Part model, mm, in its own coordinate system. A direction names the side the tool comes from. Coordinates: 2 decimals unless noted, no trailing zeros. Write each loop counter-clockwise with the first axis right and the second up, starting at its lowest first coordinate (ties: lowest second). Pieces come first, ordered by that corner, then holes. Notation, with made-up numbers: (26.5, 80) - (38.5, 80) arc R28 ccw to (38.5, 110) - close; hole circle Ø10 at (78.5, -2). An arc over 180 degrees is marked (long way). Use one line per item in the form item = value. Start each with the question number.
Autodesk Inventor part; units mm, degrees
ref_plane "YZ Plane" through (0, 0, 0) normal (1, 0, 0) x (0, 1, 0)
ref_plane "XZ Plane" through (0, 0, 0) normal (0, 1, 0) x (-1, 0, 0)
ref_plane "XY Plane" through (0, 0, 0) normal (0, 0, 1) x (1, 0, 0)
sketch "Sketch1" plane through (0, 0, 0) normal (0, 1, 0) x (-1, 0, 0)
  line L0 (-20, 40) -> (20, 40)
  line L1 (20, 40) -> (20, -40)
  line L2 (20, -40) -> (-20, -40)
  line L3 (-20, -40) -> (-20, 40)
  arc A0 (20, 14.9917) -> (20, -14.9917) centre (20.5, 0) ccw
  point P0 (0, 0)
  dimension "d0" = 80
  dimension "d1" = 40
  dimension "d2" = 40
  dimension "d3" = 20
  dimension "d4" = 30
  dimension "d22" = 0.5
extrude "Extrusion1" add sketch "Sketch1" along normal blind 20 contours L0 L1 A0 L2 L3
sketch "Sketch2" plane through (20, 0, 40) normal (1, 0, 0) x (0, 0, -1)
  line L0 (0, 0) -> (80, 0)
  line L1 (80, 0) -> (80, 20)
  line L2 (0, 20) -> (80, 20)
  line L3 (0, 0) -> (0, 20)
  point P0 (40, 0)
  point P1 (10, 10)
  point P2 (70, 10)
  dimension "d8" = 10
  dimension "d9" = 10
  dimension "d10" = 10
  dimension "d11" = 10
hole "Hole1" at (20, 10, 30) at (20, 10, -30) direction (-1, 0, 0) diameter 6 end through all
sketch "Sketch3" plane through (0, 20, 0) normal (0, 1, 0) x (1, 0, 0)
  line L0 (20, -40) -> (20, 40)
  line L1 (20, 40) -> (-20, 40)
  line L2 (-20, 40) -> (-20, 14.9917)
  arc A0 (-20, -14.9917) -> (-20, 14.9917) centre (-20.5, 0) ccw
  line L3 (-20, -14.9917) -> (-20, -40)
  line L4 (-20, -40) -> (20, -40)
  line L5 (20, -17.75) -> (2.75, -17.75)
  line L6 (2.75, -17.75) -> (2.75, 17.75)
  line L7 (2.75, 17.75) -> (20, 17.75)
  point P0 (0, 0)
  dimension "d19" = 17.25
  dimension "d20" = 35.5
  dimension "d21" = 17.75
extrude "Extrusion2" cut sketch "Sketch3" against normal through all contours L5 L6 L7 L0
fillet "Fillet1" radius 3 4 edges at (0, 20, 40) (0, 0, 40) (0, 20, -40) (0, 0, -40)
properties part number "3DP_ASA_Balcony_Mounting_Clamp_Mid"
Q1. Slice it at D-D (y = 14.5). List the corners of the cut face in (x, z), plus the area to 3 significant figures.
Q2. Drill centre lines: probe 1 along Z at (x, y) = (-2, 10); probe 2 along Z at (x, y) = (12, 10); probe 3 along Y at (x, z) = (-1.5, 30). Where is each one in solid material? Low to high.
Q3. Slice it at C-C (z = 30). List the corners of the cut face in (x, y), plus the area to 3 significant figures.
Q4. Which spindle directions (+Z, -Z, +X, -X, +Y, -Y) get a long thin tool onto all of the face, cutting with end or side? Do faces 4 (the flat face through (11, 10, 17.75)), 5 (the flat face through (-20, 7.6, 27.7)). Say none if no direction does.
Q5. Slice it at A-A (x = 7). List the corners of the cut face in (y, z).
Q6. Mould opens along Y. For faces 1 (the flat face through (2.75, 10, 0)), 2 (the cylindrical face through (0.28, 19.1, -39.14)), 3 (the cylindrical face through (0, 10, 33)) say: released by +Y, released by -Y, zero draft, split by the parting line, or undercut.
Q7. Slice it at B-B (y = 10). List the corners of the cut face in (x, z).
Q8. Pin check, flat tips, straight feed: P1, Ø10, axis at y = 15.5, z = -7, coming from the -X side; P2, Ø5, axis at y = 10, z = 30, coming from the +X side; P3, Ø6, axis at y = 8, z = 7, coming from the +X side. Stop position of each tip, or through.
Solution:
q1.outline = (-20, -40) - (20, -40) - (20, -17.75) - (2.75, -17.75) - (2.75, 17.75) - (20, 17.75) - (20, 40) - (-20, 40) - (-20, 14.99) arc R15 cw to (-20, -14.99) - close
q1.area = 2,250 mm2
q2.probe_1 = -40 to -33, -27 to 27, 33 to 40
q2.probe_2 = -40 to -33, -27 to -17.75, 17.75 to 27, 33 to 40
q2.probe_3 = 0 to 7, 13 to 20
q3.outline = (-20, 0) - (20, 0) - (20, 7) - (-20, 7) - close; (-20, 13) - (20, 13) - (20, 20) - (-20, 20) - close
q3.area = 560 mm2
q4.face_4 = +X, +Y, -Y
q4.face_5 = +Z, -Z, -X, +Y, -Y
q5.outline = (0, -37) arc R3 ccw to (3, -40) - (17, -40) arc R3 ccw to (20, -37) - (20, -17.75) - (0, -17.75) - close; (0, 17.75) - (20, 17.75) - (20, 37) arc R3 ccw to (17, 40) - (3, 40) arc R3 ccw to (0, 37) - close; hole circle Ø6 at (10, -30); hole circle Ø6 at (10, 30)
q6.face_1 = zero draft
q6.face_2 = released by +Y
q6.face_3 = undercut
q7.outline = (-20, -40) - (20, -40) - (20, -33) - (-20, -33) - close; (-20, -27) - (20, -27) - (20, -17.75) - (2.75, -17.75) - (2.75, 17.75) - (20, 17.75) - (20, 27) - (-20, 27) - (-20, 14.99) arc R15 cw to (-20, -14.99) - close; (-20, 33) - (20, 33) - (20, 40) - (-20, 40) - close
q8.P1 = -11.5
q8.P2 = through
q8.P3 = 2.75
